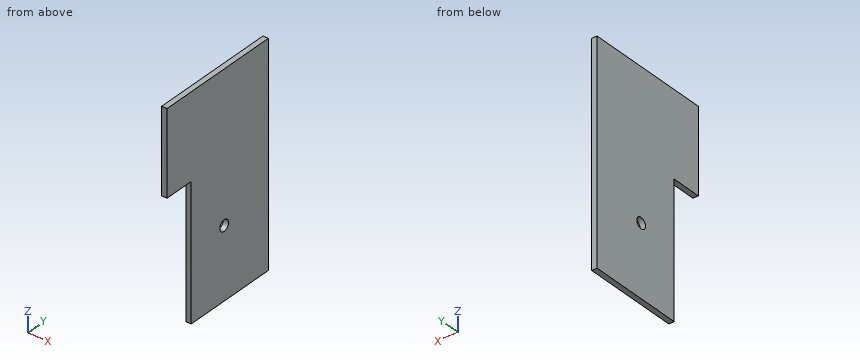
Autodesk Inventor part; units mm, degrees
ref_plane "YZ Plane" through (0, 0, 0) normal (1, 0, 0) x (0, 1, 0)
ref_plane "XZ Plane" through (0, 0, 0) normal (0, 1, 0) x (-1, 0, 0)
ref_plane "XY Plane" through (0, 0, 0) normal (0, 0, 1) x (1, 0, 0)
sketch "Sketch1" plane through (0, 0, 0) normal (1, 0, 0) x (0, 1, 0)
  line L0 (0, 12.6) -> (0, -75.6)
  line L1 (-44.1, 0) -> (7.35, 0)
  line L2 (0, 0) -> (0, -63)
  line L3 (0, -63) -> (-28, -63)
  line L4 (-28, -63) -> (-28, -24.33)
  line L5 (-28, -24.33) -> (-36.75, -24.33)
  line L6 (-36.75, -24.33) -> (-36.75, 0)
  line L7 (-36.75, 0) -> (0, 0)
  circle A0 centre (-16, -42.5) radius 1.575 construction
  dimension "d0" = 63
  dimension "d1" = 28
  dimension "d2" = 36.75
  dimension "d3" = 24.33
  dimension "d4" = 42.5
  dimension "d5" = 16
  dimension "d6" = 3.15
extrude "Extrusion1" add sketch "Sketch1" against normal blind 1.55
hole "Hole1" at (0, -16, -42.5) direction (-1, 0, 0) diameter 3.15 end through all
properties part number "J010361" material "FR4"
Build history of the part. All positions in model axes, mm. Round coordinates to 2 decimals unless told otherwise and drop trailing zeros. Write each loop counter-clockwise with the first axis right and the second up, starting at its lowest first coordinate (ties: lowest second). Pieces come first, ordered by that corner, then holes. Notation, with made-up numbers: M 77.25,74.5 L 114.25,74.5 A23 ccw 114.25,92.5 Z; hole C 24.25,13.25 d3. An arc over 180 degrees is marked long. Use CSV: the item, a comma, the result in double quotes.
1. Saw through at D-D (z = -30). Give the cut face in (x, y), plus the area to 3 significant figures.
Reply:
outline,"M -1.55,-28 L 0,-28 L 0,0 L -1.55,0 Z"
area,"43.4 mm²"
2. Saw through at B-B (z = -42.5). Give the cut face in (x, y) (3 decimals), plus the area to 3 significant figures.
Reply:
outline,"M -1.55,-28 L 0,-28 L 0,-17.575 L -1.55,-17.575 Z; M -1.55,-14.425 L 0,-14.425 L 0,0 L -1.55,0 Z"
area,"38.5 mm²"
3. Wall check: probe 1 along Z at (x, y) = (-0.35, -16) (3 decimals); probe 2 along Y at (x, z) = (-0.95, -42.5) (3 decimals); probe 3 along Z at (x, y) = (-0.9, -30.5). Give the ranges that are in metal, low to high. Write a range as from..to.
Reply:
probe 1,"z = -63..-44.075, -40.925..0"
probe 2,"y = -28..-17.575, -14.425..0"
probe 3,"z = -24.33..0"
4. Saw through at C-C (x = -1.25). Give the cut face in (y, z) (3 decimals).
Reply:
outline,"M -36.75,-24.33 L -28,-24.33 L -28,-63 L 0,-63 L 0,0 L -36.75,0 Z; hole C -16,-42.5 d3.15"
5. Flat gauge pin, fed straight in: pin 1 (0.8 mm diameter, centred on x = -1, z = -48.5, fed in from -Y). Where does the tip first touch, or does it go through?
Reply:
pin 1,"stops at y = -28"
6. Saw through at A-A (y = -16). Give the cut face in (x, z) (3 decimals).
Reply:
outline,"M -1.55,-63 L 0,-63 L 0,-44.075 L -1.55,-44.075 Z; M -1.55,-40.925 L 0,-40.925 L 0,0 L -1.55,0 Z"
